The listing builds one solid part. Answer for the finished solid, in the listing's coordinates (mm). Round coordinates to 2 decimals unless told otherwise and drop trailing zeros. Order: outer loops, then holes, each group sorted by start corner. A loop starts at its lowest first (then second) coordinate and runs counter-clockwise, first axis right, second up. Notation, with made-up numbers: (9, 27.5) -> (41, 27.5) arc R21 ccw to (41, 48.5) -> close; hole circle Ø6 at (69, 33). An arc over 180 degrees is marked (long way). Return JSON: item names as keys, results as strings. Group by question number.
(1) The part is cut by section A-A (x = -54). Determine the outline of the cut face in (y, z), plus the area to 3 significant figures.
(2) Consider line 1 (Z direction, x = 61, y = 0.2); line 2 (X direction, y = 3.15, z = 44); line 3 (Z direction, x = -19, y = 3.7). Determine where each line is inside the solid, lowest interval first. Write a range as [from, to].
(3) The part is cut by section D-D (x = -3). Determine the outline of the cut face in (y, z), plus the area to 3 significant figures.
(4) The part is cut by section B-B (z = 44.5). Determine the outline of the cut face in (x, y), plus the area to 3 significant figures.
(5) The part is cut by section C-C (y = 1.75). Count the separate pieces of the cut face and the enclosed holes in it, plus the area to 3 significant figures.
(6) This flat-tipped pin is pushed along its axis until it touches: pin 1 (1.2 mm diameter, centred on x = -15, y = 2, fed in from +Z). Where does it stop, or does it pass through?
from build123d import *

# Parameters (mm, degrees)
EXTRUDE_1_DEPTH     = 4
SKETCH_2_W          = 10.5
SKETCH_2_H          = 4.5
CUT_EXTRUDE_1_DEPTH = 147.512735554


with BuildPart() as part:
    # Эскиз1 → Бобышка-Вытянуть1 (new body)
    with BuildSketch(Plane(origin=(0, 0, 0), x_dir=(1, 0, 0), z_dir=(0, 1, 0))):
        Polygon((-135, -16.788922156), (-135, -56.788922156), (-105, -56.788922156), (-105, -16.788922156), (55, -16.788922156), (55, -56.788922156), (85, -56.788922156), (85, -16.788922156), (85, 3.211077844), (-135, 3.211077844), align=None)
    extrude(amount=EXTRUDE_1_DEPTH)

    # Эскиз2 → Вырез-Вытянуть1 (cut, through all)
    with BuildSketch(Plane(origin=(0, 0, 0), x_dir=(1, 0, 0), z_dir=(0, 1, 0))):
        with Locations((-115, -11.788922156)):
            Rectangle(SKETCH_2_W, SKETCH_2_H)
        with Locations((-95, -11.788922156)):
            Rectangle(SKETCH_2_W, SKETCH_2_H)
        with Locations((-75, -11.788922156)):
            Rectangle(SKETCH_2_W, SKETCH_2_H)
        with Locations((-55, -11.788922156)):
            Rectangle(SKETCH_2_W, SKETCH_2_H)
        with Locations((-35, -11.788922156)):
            Rectangle(SKETCH_2_W, SKETCH_2_H)
        with Locations((-15, -11.788922156)):
            Rectangle(SKETCH_2_W, SKETCH_2_H)
        with Locations((5, -11.788922156)):
            Rectangle(SKETCH_2_W, SKETCH_2_H)
        with Locations((25, -11.788922156)):
            Rectangle(SKETCH_2_W, SKETCH_2_H)
        with Locations((45, -11.788922156)):
            Rectangle(SKETCH_2_W, SKETCH_2_H)
        with Locations((65, -11.788922156)):
            Rectangle(SKETCH_2_W, SKETCH_2_H)
    extrude(amount=CUT_EXTRUDE_1_DEPTH, mode=Mode.SUBTRACT)


solid = part.part
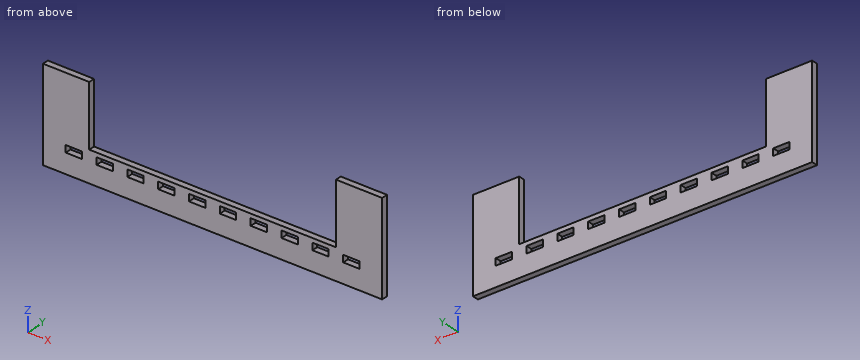
Answer below:
{
 "1": {"outline": "(0, -3.21) -> (4, -3.21) -> (4, 9.54) -> (0, 9.54) -> close; (0, 14.04) -> (4, 14.04) -> (4, 16.79) -> (0, 16.79) -> close", "area": "62.0 mm²"},
 "2": {"line 1": "z = [-3.21, 9.54], [14.04, 56.79]", "line 2": "x = [-135, -105], [55, 85]", "line 3": "z = [-3.21, 9.54], [14.04, 16.79]"},
 "3": {"outline": "(0, -3.21) -> (4, -3.21) -> (4, 16.79) -> (0, 16.79) -> close", "area": "80.0 mm²"},
 "4": {"outline": "(-135, 0) -> (-105, 0) -> (-105, 4) -> (-135, 4) -> close; (55, 0) -> (85, 0) -> (85, 4) -> (55, 4) -> close", "area": "240 mm²"},
 "5": {"separate pieces": "1", "enclosed holes": "10", "area": "6,330 mm²"},
 "6": {"pin 1": "stops at z = 16.79"}
}
